Can you work these out from the model? Positions are in its coordinate system, mm. A direction names the side the tool comes from. Give positions to 0.01 mm unless a question says otherwise; leave off trailing zeros. Loops run counter-clockwise (first coordinate to the right, second up) from the corner with the lowest first, then second, coordinate; pieces in that order, holes last. Notation, with made-up numbers: (71.25, -35) - (125.25, -35) arc R25 cw to (125.25, -7) - close; hole circle Ø10 at (10.25, 36.5). An arc over 180 degrees is marked (long way). Answer in a Markdown table with one row per item.
from build123d import *

# Parameters (mm, degrees)
SKETCH1_R           = 1
SKETCH1_R_2         = 1.0000000000000018
BOSS_EXTRUDE1_DEPTH = 2.5
SKETCH2_R           = 2.7499999999999996
CUT_EXTRUDE1_DEPTH  = 2.5
CHAMFER1_SIZE       = 5
CHAMFER1_SIZE2      = 1.819851171331016
CUT_EXTRUDE2_DEPTH  = 2.5
CHAMFER2_SIZE       = 0.5
CHAMFER3_SIZE       = 2
SKETCH4_W           = 2.9999999999999982
SKETCH4_H           = 2
CUT_EXTRUDE3_DEPTH  = 2.5
CHAMFER4_SIZE       = 2
CHAMFER4_SIZE2      = 0.7279404685324065
FILLET1_R           = 1


with BuildPart() as part:
    # Sketch1 → Boss-Extrude1 (new body)
    with BuildSketch(Plane.XY):
        with BuildLine():
            Line((21.499999999999993, -26.999999999999996), (-21.499999999999993, -26.999999999999996))
            ThreePointArc((-21.499999999999993, -26.999999999999996), (-22.207106781186546, -26.707106781186543), (-22.5, -25.99999999999999))
            Line((-22.5, -25.99999999999999), (-22.5, 25.99999999999999))
            ThreePointArc((-22.5, 25.99999999999999), (-22.207106781186546, 26.707106781186543), (-21.499999999999993, 26.999999999999996))
            Line((-21.499999999999993, 26.999999999999996), (21.499999999999993, 26.999999999999996))
            ThreePointArc((21.499999999999993, 26.999999999999996), (22.207106781186546, 26.707106781186543), (22.5, 25.99999999999999))
            Line((22.5, 25.99999999999999), (22.5, -25.99999999999999))
            ThreePointArc((22.5, -25.99999999999999), (22.207106781186546, -26.707106781186543), (21.499999999999993, -26.999999999999996))
        make_face()
        with Locations((-10.018444645439217, 23.665000000000006)):
            Circle(SKETCH1_R, mode=Mode.SUBTRACT)
        with Locations((-17, -22.000000000000007)):
            Circle(SKETCH1_R_2, mode=Mode.SUBTRACT)
        with Locations((17, -22.000000000000004)):
            Circle(SKETCH1_R_2, mode=Mode.SUBTRACT)
    extrude(amount=BOSS_EXTRUDE1_DEPTH)

    # Sketch2 → Cut-Extrude1 (cut)
    with BuildSketch(Plane.XY.offset(2.5)):
        with Locations((0, 14.599999999999996)):
            Circle(SKETCH2_R)
    extrude(amount=-CUT_EXTRUDE1_DEPTH, mode=Mode.SUBTRACT)

    # Chamfer1
    chamfer1_edges = [part.edges().sort_by_distance(p)[0] for p in [
        (-2.7499999999999996, 14.599999999999996, 2.5),
    ]]
    chamfer1_side = [part.faces().sort_by_distance(p)[0] for p in [
        (0.01313623413448006, -0.11811006320101064, 2.5),
    ]]
    chamfer(chamfer1_edges, length=CHAMFER1_SIZE, length2=CHAMFER1_SIZE2, reference=chamfer1_side[0])

    # Sketch3 → Cut-Extrude2 (cut)
    with BuildSketch(Plane.XY.offset(2.5)):
        with BuildLine():
            Line((-12.5, 2), (12.5, 2.0000000000000053))
            ThreePointArc((12.5, 2.0000000000000053), (13.5, 1.0000000000000036), (12.5, 4.34e-15))
            Line((12.5, 4.34e-15), (-12.5, 0))
            ThreePointArc((-12.5, 0), (-13.5, 1.0000000000000002), (-12.5, 2))
        make_face()
        with BuildLine():
            Line((-12.5, -2), (12.5, -2))
            ThreePointArc((12.5, -2), (13.5, -3), (12.5, -4))
            Line((12.5, -4), (-12.5, -4))
            ThreePointArc((-12.5, -4), (-13.5, -3), (-12.5, -2))
        make_face()
        with BuildLine():
            Line((-12.5, -6.000000000000001), (12.5, -6.000000000000001))
            ThreePointArc((12.5, -6.000000000000001), (13.5, -7), (12.5, -8))
            Line((12.5, -8), (-12.5, -8))
            ThreePointArc((-12.5, -8), (-13.5, -7), (-12.5, -6.000000000000001))
        make_face()
        with BuildLine():
            Line((-12.5, -9.999999999999998), (12.5, -9.999999999999998))
            ThreePointArc((12.5, -9.999999999999998), (13.5, -11), (12.5, -12))
            Line((12.5, -12), (-12.5, -12))
            ThreePointArc((-12.5, -12), (-13.500000000000002, -11), (-12.5, -9.999999999999998))
        make_face()
    extrude(amount=-CUT_EXTRUDE2_DEPTH, mode=Mode.SUBTRACT)

    # Chamfer2
    chamfer2_edges = [part.edges().sort_by_distance(p)[0] for p in [
        (-13.5, 0.9999999999999999, 0),
        (0, 2.0000000000000027, 0),
        (13.5, 1.0000000000000049, 0),
        (0, 2.17e-15, 0),
        (-13.5, 0.9999999999999999, 2.5),
        (0, 2.17e-15, 2.5),
        (13.5, 1.0000000000000049, 2.5),
        (0, 2.0000000000000027, 2.5),
        (-13.5, -3, 0),
        (0, -2, 0),
        (13.5, -3, 0),
        (0, -4, 0),
        (-13.5, -3, 2.5),
        (0, -4, 2.5),
        (13.5, -3, 2.5),
        (0, -2, 2.5),
        (-13.5, -7, 0),
        (0, -6.000000000000001, 0),
        (13.5, -7, 0),
        (0, -8, 0),
        (-13.5, -7, 2.5),
        (0, -8, 2.5),
        (13.5, -7, 2.5),
        (0, -6.000000000000001, 2.5),
        (-13.500000000000002, -11, 0),
        (0, -9.999999999999998, 0),
        (13.5, -11, 0),
        (0, -12, 0),
        (-13.500000000000002, -11, 2.5),
        (0, -12, 2.5),
        (13.5, -11, 2.5),
        (0, -9.999999999999998, 2.5),
    ]]
    chamfer(chamfer2_edges, length=CHAMFER2_SIZE)

    # Chamfer3
    chamfer3_edges = [part.edges().sort_by_distance(p)[0] for p in [
        (-11.018444645439217, 23.665000000000006, 2.5),
        (-18, -22.000000000000007, 2.5),
        (15.999999999999998, -22.000000000000004, 2.5),
    ]]
    chamfer(chamfer3_edges, length=CHAMFER3_SIZE)

    # Sketch4 → Cut-Extrude3 (cut)
    with BuildSketch(Plane.XY.offset(2.5)):
        with Locations((-16.7, 17.799999999999997)):
            Rectangle(SKETCH4_W, SKETCH4_H)
        with Locations((16.7, 17.799999999999997)):
            Rectangle(SKETCH4_W, SKETCH4_H)
    extrude(amount=-CUT_EXTRUDE3_DEPTH, mode=Mode.SUBTRACT)

    # Chamfer4
    chamfer4_edges = [part.edges().sort_by_distance(p)[0] for p in [
        (-15.200000000000001, 17.799999999999997, 2.5),
        (-16.7, 18.799999999999997, 2.5),
        (-18.2, 17.799999999999997, 2.5),
        (-16.7, 16.799999999999997, 2.5),
        (18.2, 17.799999999999997, 2.5),
        (16.7, 18.799999999999997, 2.5),
        (15.200000000000001, 17.799999999999997, 2.5),
        (16.7, 16.799999999999997, 2.5),
    ]]
    chamfer4_side = [part.faces().sort_by_distance(p)[0] for p in [
        (0, -26.297077529168398, 2.5),
    ]]
    chamfer(chamfer4_edges, length=CHAMFER4_SIZE, length2=CHAMFER4_SIZE2, reference=chamfer4_side[0])

    # Fillet1
    # the kernel refuses this fillet: 1 mm, written as the material it takes off along each edge
    with BuildSketch(Plane(origin=(21.499999999999996, -25.999999999999993, 2.5), x_dir=(1, 3.55e-15, 0), z_dir=(-3.55e-15, 1, 0))) as fillet1_piece_1:
        with BuildLine():
            CenterArc((1.0000000000000036 - FILLET1_R, FILLET1_R), FILLET1_R, 270, 90)
            Line((1.0000000000000036, FILLET1_R), (1.0000000000000036, 0))
            Line((1.0000000000000036, 0), (1.0000000000000036 - FILLET1_R, 0))
        make_face()
    revolve(axis=Axis((21.499999999999996, -25.999999999999993, 2.5), (0, 0, -1)), revolution_arc=90.00000000000041, mode=Mode.SUBTRACT)
    with BuildSketch(Plane(origin=(22.5, 25.99999999999999, 2.5), x_dir=(-1, 0, 0), z_dir=(0, -1, 0)), Plane(origin=(-22.5, -25.99999999999999, 2.5), x_dir=(1, 0, 0), z_dir=(0, 1, 0))) as fillet1_piece_2:
        with BuildLine():
            CenterArc((FILLET1_R, FILLET1_R), FILLET1_R, 180, 90)
            Line((0, FILLET1_R), (0, 0))
            Line((0, 0), (FILLET1_R, 0))
        make_face()
    extrude(amount=51.99999999999998, mode=Mode.SUBTRACT)
    with BuildSketch(Plane(origin=(21.499999999999996, 25.999999999999993, 2.5), x_dir=(-3.55e-15, 1, 0), z_dir=(-1, -3.55e-15, 0))) as fillet1_piece_3:
        with BuildLine():
            CenterArc((1.0000000000000036 - FILLET1_R, FILLET1_R), FILLET1_R, 270, 90)
            Line((1.0000000000000036, FILLET1_R), (1.0000000000000036, 0))
            Line((1.0000000000000036, 0), (1.0000000000000036 - FILLET1_R, 0))
        make_face()
    revolve(axis=Axis((21.499999999999996, 25.999999999999993, 2.5), (0, 0, -1)), revolution_arc=90.00000000000041, mode=Mode.SUBTRACT)
    with BuildSketch(Plane(origin=(-21.499999999999993, 26.999999999999996, 2.5), x_dir=(0, -1, 0), z_dir=(1, 0, 0)), Plane(origin=(21.499999999999993, -26.999999999999996, 2.5), x_dir=(0, 1, 0), z_dir=(-1, 0, 0))) as fillet1_piece_4:
        with BuildLine():
            CenterArc((FILLET1_R, FILLET1_R), FILLET1_R, 180, 90)
            Line((0, FILLET1_R), (0, 0))
            Line((0, 0), (FILLET1_R, 0))
        make_face()
    extrude(amount=42.999999999999986, mode=Mode.SUBTRACT)
    with BuildSketch(Plane(origin=(-21.499999999999996, 25.999999999999993, 2.5), x_dir=(-1, -3.55e-15, 0), z_dir=(3.55e-15, -1, 0))) as fillet1_piece_5:
        with BuildLine():
            CenterArc((1.0000000000000036 - FILLET1_R, FILLET1_R), FILLET1_R, 270, 90)
            Line((1.0000000000000036, FILLET1_R), (1.0000000000000036, 0))
            Line((1.0000000000000036, 0), (1.0000000000000036 - FILLET1_R, 0))
        make_face()
    revolve(axis=Axis((-21.499999999999996, 25.999999999999993, 2.5), (0, 0, -1)), revolution_arc=90.00000000000041, mode=Mode.SUBTRACT)
    with BuildSketch(Plane(origin=(-21.499999999999996, -25.999999999999993, 2.5), x_dir=(3.55e-15, -1, 0), z_dir=(1, 3.55e-15, 0))) as fillet1_piece_6:
        with BuildLine():
            CenterArc((1.0000000000000036 - FILLET1_R, FILLET1_R), FILLET1_R, 270, 90)
            Line((1.0000000000000036, FILLET1_R), (1.0000000000000036, 0))
            Line((1.0000000000000036, 0), (1.0000000000000036 - FILLET1_R, 0))
        make_face()
    revolve(axis=Axis((-21.499999999999996, -25.999999999999993, 2.5), (0, 0, -1)), revolution_arc=90.00000000000041, mode=Mode.SUBTRACT)


solid = part.part
Q1. If I drill on line 1 (Y direction, x = -17, z = 0.35); line 2 (X direction, y = -22, z = 0.35); line 3 (Y direction, x = -6, z = 1.05), over which ranges is the centre line in solid material (lowest first)? Write a range as [from, to].
Checked values:
| item | result |
|---|---|
| line 1 | y = [-27, -23], [-21, 16.8], [18.8, 27] |
| line 2 | x = [-22.5, -18], [-16, 16], [18, 22.5] |
| line 3 | y = [-27, -12], [-10, -8], [-6, -4], [-2, 0], [2, 27] |
Q2. For pin 1 (7 mm diameter, centred on x = 0, y = 14.6, fed in from +Z), with a flat end and sliding along its axis, tell me the tip position at first contact or that it passes through.
Checked values:
| item | result |
|---|---|
| pin 1 | stops at z = 0.95 |
Q3. Imagine slicing it at A-A, the plane y = -22. Write out the boundary of the cut face in (x, z), and give its area (3 significant figures).
Checked values:
| item | result |
|---|---|
| outline | (-22.5, 0) - (-18, 0) - (-18, 0.5) - (-20, 2.5) - (-21.5, 2.5) arc R1 ccw to (-22.5, 1.5) - close; (-16, 0) - (16, 0) - (16, 0.5) - (14, 2.5) - (-14, 2.5) - (-16, 0.5) - close; (18, 0) - (22.5, 0) - (22.5, 1.5) arc R1 ccw to (21.5, 2.5) - (20, 2.5) - (18, 0.5) - close |
| area | 94.1 mm² |
Q4. Imagine slicing it at C-C, the plane x = 0. Count the separate pieces of the cut face and the enclosed holes in it, and give its area (3 significant figures).
Checked values:
| item | result |
|---|---|
| separate pieces | 6 |
| enclosed holes | 0 |
| area | 89.7 mm² |
Q5. Imagine slicing it at B-B, the plane y = -3. Write out the boundary of the cut face in (x, z).
Checked values:
| item | result |
|---|---|
| outline | (-22.5, 0) - (-14, 0) - (-13.5, 0.5) - (-13.5, 2) - (-14, 2.5) - (-21.5, 2.5) arc R1 ccw to (-22.5, 1.5) - close; (13.5, 0.5) - (14, 0) - (22.5, 0) - (22.5, 1.5) arc R1 ccw to (21.5, 2.5) - (14, 2.5) - (13.5, 2) - close |
Q6. On a 3-axis mill with a long thin cutter (end or side, diameter ignored), from which of +Z, -Z, +X, -X, +Y, -Y can I reach the whole of each face in a straight line? I mean faces 1 (the face through (-16.749, 20.008, 2.212)), 2 (the face through (-13.5, 1, 1.3)). Say none if no direction works.
Checked values:
| item | result |
|---|---|
| face 1 | +Z |
| face 2 | +Z, -Z |
